```python
from build123d import *

# Parameters (mm, degrees)
F1_DEPTH  = 190
F2_T      = -2
F3_W      = 51
F3_H      = 19
F3_W_2    = 97
F3_H_2    = 40
F4_DEPTH  = 2
F5_R      = 3.5
F5_R_2    = 6
F6_DEPTH  = 2
F7_W      = 9.5
F7_H      = 11.5
F7_W_2    = 13.1
F7_H_2    = 11.7
F8_DEPTH  = 2
F9_W      = 22
F9_H      = 3.5
F10_DEPTH = 2
F11_R     = 1.75
F11_R_2   = 0.75
F12_DEPTH = 4.5
F13_R     = 3
F13_R_2   = 2
F14_DEPTH = 4.5
F15_R     = 2
F16_DEPTH = 8
F17_R     = 0.5


with BuildPart() as f1:
    # F0 (on Right) → F1 (new body)
    with BuildSketch(Plane.YZ):
        Polygon((0, 30), (0, 0), (90.9326673974, 0), (90.9326673974, 82.5), align=None)
    extrude(amount=F1_DEPTH)

    # F2
    f2_openings = [f1.faces().sort_by_distance(p)[0] for p in [
        (95, 45.466334, 0),
    ]]
    offset(amount=F2_T, openings=f2_openings)

    # F3 (on face) → F4 (cut)
    with BuildSketch(Plane(origin=(0, -12.9903810568, 22.5), x_dir=(1, 0, 0), z_dir=(0, -0.5, 0.8660254038))):
        with Locations((35.5, 100.5)):
            Rectangle(F3_W, F3_H)
        with Locations((58.5, 51)):
            Rectangle(F3_W_2, F3_H_2)
    extrude(amount=-F4_DEPTH, mode=Mode.SUBTRACT)

    # F5 (on face) → F6 (cut)
    with BuildSketch(Plane(origin=(0, -12.9903810568, 22.5), x_dir=(1, 0, 0), z_dir=(0, -0.5, 0.8660254038))):
        with Locations((122.5, 33)):
            Circle(F5_R)
        with Locations((147.5, 33)):
            Circle(F5_R_2)
        with Locations((172.5, 33)):
            Circle(F5_R_2)
    extrude(amount=-F6_DEPTH, mode=Mode.SUBTRACT)

    # F7 (on face) → F8 (cut)
    with BuildSketch(Plane.YZ.offset(190)):
        with Locations((66.1826673974, 10.5)):
            Rectangle(F7_W, F7_H)
        with Locations((35.7826673974, 10.6)):
            Rectangle(F7_W_2, F7_H_2)
    extrude(amount=-F8_DEPTH, mode=Mode.SUBTRACT)

    # F9 (on face) → F10 (cut)
    with BuildSketch(Plane(origin=(0, -12.9903810568, 22.5), x_dir=(1, 0, 0), z_dir=(0, -0.5, 0.8660254038))):
        with Locations((159, 62.75)):
            Rectangle(F9_W, F9_H)
    extrude(amount=-F10_DEPTH, mode=Mode.SUBTRACT)

    # F11 (on face) → F12 (join)
    with BuildSketch(Plane(origin=(0, -12.9903810568, 22.5), x_dir=(1, 0, 0), z_dir=(0, -0.5, 0.8660254038))):
        with Locations((14, 112)):
            Circle(F11_R)
        with Locations((14, 112)):
            Circle(F11_R_2, mode=Mode.SUBTRACT)
        with Locations((14, 89)):
            Circle(F11_R)
        with Locations((14, 89)):
            Circle(F11_R_2, mode=Mode.SUBTRACT)
        with Locations((57, 112)):
            Circle(F11_R)
        with Locations((57, 112)):
            Circle(F11_R_2, mode=Mode.SUBTRACT)
        with Locations((57, 89)):
            Circle(F11_R)
        with Locations((57, 89)):
            Circle(F11_R_2, mode=Mode.SUBTRACT)
    extrude(amount=-F12_DEPTH)

    # F13 (on face) → F14 (join)
    with BuildSketch(Plane(origin=(0, -12.9903810568, 22.5), x_dir=(1, 0, 0), z_dir=(0, -0.5, 0.8660254038))):
        with Locations((13, 78)):
            Circle(F13_R)
        with Locations((13, 78)):
            Circle(F13_R_2, mode=Mode.SUBTRACT)
        with Locations((104, 78)):
            Circle(F13_R)
        with Locations((104, 78)):
            Circle(F13_R_2, mode=Mode.SUBTRACT)
        with Locations((104, 24)):
            Circle(F13_R)
        with Locations((104, 24)):
            Circle(F13_R_2, mode=Mode.SUBTRACT)
        with Locations((13, 24)):
            Circle(F13_R)
        with Locations((13, 24)):
            Circle(F13_R_2, mode=Mode.SUBTRACT)
    extrude(amount=-F14_DEPTH)

    # F15 (on face) → F16 (join)
    with BuildSketch(Plane(origin=(0, 0, 0), x_dir=(1, 0, 0), z_dir=(0, 0, -1))):
        with Locations((3, -3)):
            Circle(F15_R)
        with Locations((3, -87.9326673974)):
            Circle(F15_R)
        with Locations((187, -3)):
            Circle(F15_R)
        with Locations((187, -87.9326673974)):
            Circle(F15_R)
    extrude(amount=-F16_DEPTH)

    # F17
    f17_edges = [f1.edges().sort_by_distance(p)[0] for p in [
        (190, 45.466334, 56.25),
        (0, 45.466334, 56.25),
        (95, 0, 30),
        (0, 0, 15),
        (190, 90.932667, 41.25),
        (0, 90.932667, 41.25),
        (95, 90.932667, 82.5),
        (95, 88.932667, 79.035898),
        (190, 0, 15),
    ]]
    fillet(f17_edges, radius=F17_R)


solid = f1.part
```
Source: CAD feature listing. Evaluate the final solid. Frame: model axes, mm. A direction names the side the tool comes from. Coordinates: 2 decimals unless noted, no trailing zeros. Loops run counter-clockwise (first coordinate to the right, second up) from the corner with the lowest first, then second, coordinate; pieces in that order, holes last. Notation, with made-up numbers: M 68,52.5 L 123,52.5 A20 ccw 123,77.5 Z; hole C 50.25,63.25 d4. An arc over 180 degrees is marked long. Put each result on its own line as item: value. Start each with the question number.
1) Ray query, L1, parallel to X at y = 57, z = 11.5; L2, parallel to Y at x = 113, z = 13; L3, parallel to Y at x = 10.5, z = 55. Return the intervals inside material, ascending. Write a range as from..to.
2) Cut plane C-C on x = 21.5. Return the cut outline in (y, z), then the cut area to 3 significant figures.
3) Cut plane D-D on z = 20. Return the cut outline in (x, y).
4) Pull-direction query (Y, two-part tool) for faces 3 (the face through (95, 1, 0)), 4 (the face through (12.972, 8.818, 32.782)); classes: pulls with the +Y half, pulls with the -Y half, needs draft (parallel to the pull), parting line crosses it, or undercut.
5) Cut plane A-A on x = 91.5. Return the cut outline in (y, z).
6) Contact query for flat-ended pins moving along their axis: pin 1 Ø1 at (x, y) = (189, 68.5) entering from +Z; pin 2 Ø2 at (x, z) = (123, 35.5) entering from -Y; pin 3 Ø3.5 at (x, y) = (187, 88) entering from +Z. Output: stop coordinate, or through.
7) Reachability of faces 1 (the face through (0, 55, 32)), 2 (the face through (103.972, 8.818, 32.782)) from +Z, -Z, +X, -X, +Y, -Y: full face, straight path, thin tool, end or side. Return the list, or none.
8) Cut plane B-B on z = 11.5. Return the cut outline in (x, y), then the cut area to 3 significant figures.
The answers:
1. L1: x = 0..2, 188..190
1. L2: y = 0..2, 88.93..90.93
1. L3: y = 88.93..90.93
2. outline: M 0,0 L 2,0 L 2,28.85 L 14.86,36.27 L 13.86,38 L 0.25,30.14 A0.5 ccw 0,29.71 Z; M 48.5,58 L 49.5,56.27 L 66.82,66.27 L 65.82,68 Z; M 82.27,77.5 L 83.27,75.77 L 88.18,78.6 A0.5 cw 88.93,78.17 L 88.93,0 L 90.93,0 L 90.93,81.63 A0.5 ccw 90.18,82.07 Z
2. area: 308 mm²
3. outline: M 0,0.5 A0.5 ccw 0.5,0 L 189.5,0 A0.5 ccw 190,0.5 L 190,90.43 A0.5 ccw 189.5,90.93 L 0.5,90.93 A0.5 ccw 0,90.43 Z; hole M 2,2 L 188,2 L 188,88.93 L 2,88.93 Z
4. face 3: needs draft
4. face 4: undercut
5. outline: M 0,0 L 2,0 L 2,28.85 L 14.86,36.27 L 13.86,38 L 0.25,30.14 A0.5 ccw 0,29.71 Z; M 48.5,58 L 49.5,56.27 L 88.18,78.6 A0.5 cw 88.93,78.17 L 88.93,0 L 90.93,0 L 90.93,81.63 A0.5 ccw 90.18,82.07 Z
6. pin 1: stops at z = 69.84
6. pin 2: stops at y = 7.79
6. pin 3: stops at z = 81.82
7. face 1: +Z, -Z, -X, +Y, -Y
7. face 2: none
8. outline: M 0,0.5 A0.5 ccw 0.5,0 L 189.5,0 A0.5 ccw 190,0.5 L 190,29.23 L 188,29.23 L 188,2 L 2,2 L 2,88.93 L 188,88.93 L 188,70.93 L 190,70.93 L 190,90.43 A0.5 ccw 189.5,90.93 L 0.5,90.93 A0.5 ccw 0,90.43 Z; M 188,42.33 L 190,42.33 L 190,61.43 L 188,61.43 Z
8. area: 1,060 mm²
